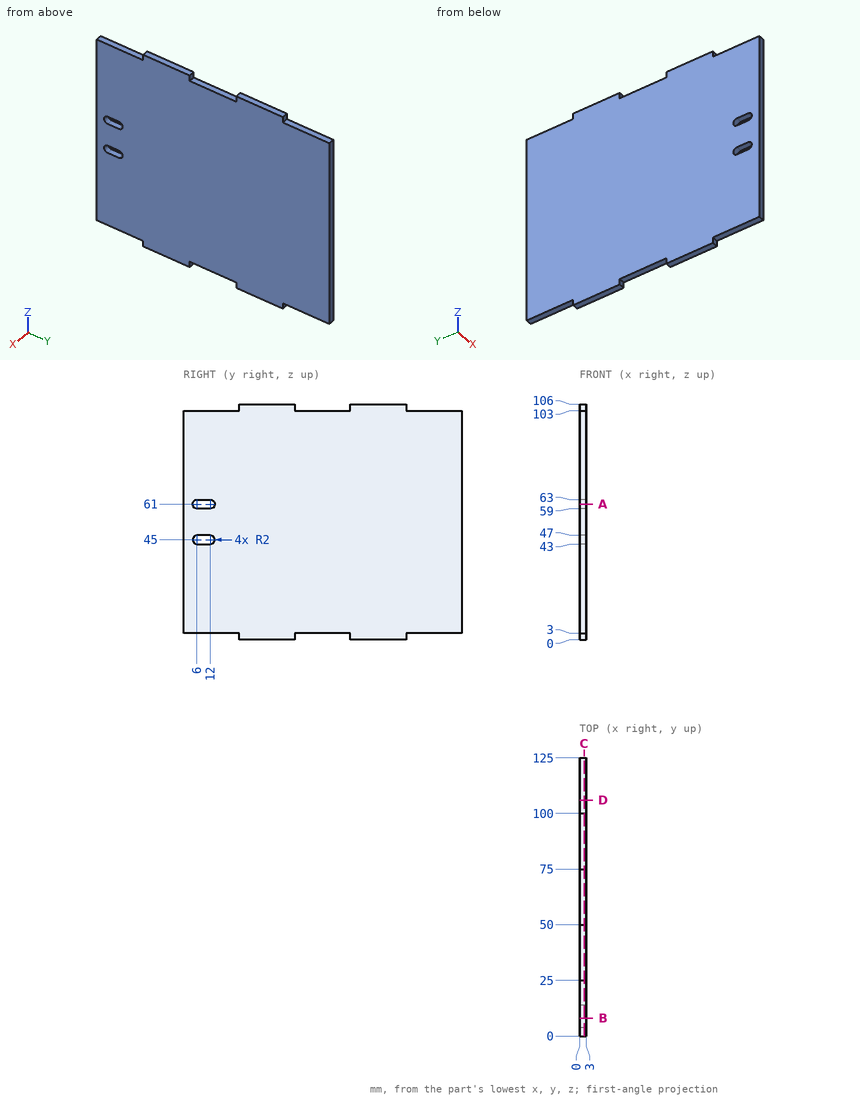
Geometry check sheet. Reference: drawing and pictorial views, mm from the part's lowest x, y, z. Give positions to 0.01 mm unless a question says otherwise; leave off trailing zeros. Write each loop counter-clockwise with the first axis right and the second up, starting at its lowest first coordinate (ties: lowest second). Pieces come first, ordered by that corner, then holes. Notation, with made-up numbers: M -1,28.5 L 32,28.5 A34 cw 32,61.5 Z; hole C 37.5,52.25 d6. An arc over 180 degrees is marked long. Put each result on its own line as item: value. Start each with the question number.
1. Section check A-A (z = 61). Record the cut outline in (x, y), and give its area (3 significant figures).
2. Scan lines: line 1 along Z through (x, y) = (2.55, 102); line 2 along Y through (x, z) = (2.05, 45.5). Record each from-to range of solid material in increasing order. Write a range as [from, to].
3. Section check C-C (x = 2). Record the cut outline in (y, z), and give its area (3 significant figures).
4. Section check B-B (y = 8). Record the cut outline in (x, z), and give its area (3 significant figures).
5. Go/stop test with flat-tipped pins: pin 1 Ø1.5 at (x, y) = (1.5, 21) entering from +Z; pin 2 Ø0.9 at (x, z) = (2, 104.5) entering from -Y; pin 3 Ø0.9 at (x, z) = (1.5, 104) entering from +Y. Record where each tip stops, or that it passes through.
6. Section check D-D (y = 106). Record the cut outline in (x, z), and give its area (3 significant figures).
Answer list:
1. outline: M 0,0 L 3,0 L 3,4 L 0,4 Z; M 0,14 L 3,14 L 3,125 L 0,125 Z
1. area: 345 mm2
2. line 1: [3, 103]
2. line 2: [0, 4.06], [13.94, 125]
3. outline: M 0,3 L 25,3 L 25,0 L 50,0 L 50,3 L 75,3 L 75,0 L 100,0 L 100,3 L 125,3 L 125,103 L 100,103 L 100,106 L 75,106 L 75,103 L 50,103 L 50,106 L 25,106 L 25,103 L 0,103 Z; hole M 6,43 L 12,43 A2 ccw 12,47 L 6,47 A2 ccw Z; hole M 6,59 L 12,59 A2 ccw 12,63 L 6,63 A2 ccw Z
3. area: 12,700 mm2
4. outline: M 0,3 L 3,3 L 3,43 L 0,43 Z; M 0,47 L 3,47 L 3,59 L 0,59 Z; M 0,63 L 3,63 L 3,103 L 0,103 Z
4. area: 276 mm2
5. pin 1: z = 103
5. pin 2: y = 25
5. pin 3: y = 100
6. outline: M 0,3 L 3,3 L 3,103 L 0,103 Z
6. area: 300 mm2
